from build123d import *

# Parameters (mm, degrees)
SZKIC1_R                    = 3
DODANIE_WYCI_GNI_CIE1_DEPTH = 2


with BuildPart() as part:
    # Szkic1 → Dodanie-wyciągnięcie1 (new body)
    with BuildSketch(Plane.XY):
        with BuildLine():
            ThreePointArc((16.690895301, 15.0061262), (12.690895301, 19.0061262), (8.690895301, 15.0061262))
            Line((8.690895301, 15.0061262), (6.71006463, -34.514640573))
            Line((6.71006463, -34.514640573), (6.690895301, -34.9938738))
            ThreePointArc((6.690895301, -34.9938738), (12.690895301, -40.9938738), (18.690895301, -34.9938738))
            Line((18.690895301, -34.9938738), (18.671725971, -34.514640573))
            Line((18.671725971, -34.514640573), (16.690895301, 15.0061262))
        make_face()
        with Locations((12.690895301, -34.9938738)):
            Circle(SZKIC1_R, mode=Mode.SUBTRACT)
        with Locations((12.690895301, 15.0061262)):
            Circle(SZKIC1_R, mode=Mode.SUBTRACT)
    extrude(amount=DODANIE_WYCI_GNI_CIE1_DEPTH)


solid = part.part
Verification items for the finished model (mm, model axes). Coordinates: 2 decimals unless noted, no trailing zeros. Order: outer loops, then holes, each group sorted by start corner. A loop starts at its lowest first (then second) coordinate and runs counter-clockwise, first axis right, second up. Notation, with made-up numbers: M -10.5,63 L 25.5,63 A22 ccw 25.5,85 Z; hole C 57,29 d4. An arc over 180 degrees is marked long. One line per item, written item: value. Start each with the question number.
Item 1: Depth check by flat-ended pin: P1, Ø7, axis at x = 12.69, y = 15.01, coming from the +Z side. Enter the tip coordinate at first touch or a pass-through.
Item 2: Sectioned sample at B-B on x = 12.75. Record the cut outline in (y, z).
Item 3: Thickness scan on probe 1 along Y at (x, z) = (12.5, 0.9); probe 2 along Y at (x, z) = (13.5, 1.25); probe 3 along X at (y, z) = (16, 0.6). Record the ranges inside material, lowest first.
Item 4: Sectioned sample at D-D on y = 10.5. Record the cut outline in (x, z).
Item 5: Sectioned sample at A-A on z = 1.6. Record the cut outline in (x, y), then the cut area to 3 significant figures.
Item 6: Mould release check, pull along Y, two halves, no side actions. Record for faces 1 (the flat face through (13, -17, 2)), 2 (the cylindrical face through (14.3, 17.54, 0.99)), 3 (the cylindrical face through (12.779, 19.005, 0.986)), 4 (the cylindrical face through (12.559, -40.992, 0.986)): pulls with the +Y half, pulls with the -Y half, needs draft (parallel to the pull), parting line crosses it, or undercut.
Item 7: Sectioned sample at C-C on y = -17. Record the cut outline in (x, z), then the cut area to 3 significant figures.
Calculated:
1. P1: z = 2
2. outline: M -40.99,0 L -37.99,0 L -37.99,2 L -40.99,2 Z; M -31.99,0 L 12.01,0 L 12.01,2 L -31.99,2 Z; M 18.01,0 L 19.01,0 L 19.01,2 L 18.01,2 Z
3. probe 1: -40.99 to -37.99, -32 to 12.01, 18 to 19
3. probe 2: -40.94 to -37.88, -32.11 to 12.12, 17.89 to 18.92
3. probe 3: 8.82 to 9.86, 15.52 to 16.57
4. outline: M 8.51,0 L 16.87,0 L 16.87,2 L 8.51,2 Z
5. outline: M 6.69,-34.99 A6 ccw 18.69,-34.99 L 16.69,15.01 A4 ccw 8.69,15.01 Z; hole C 12.69,-34.99 d6; hole C 12.69,15.01 d6
5. area: 525 mm^2
6. face 1: needs draft
6. face 2: undercut
6. face 3: pulls with the +Y half
6. face 4: pulls with the -Y half
7. outline: M 7.41,0 L 17.97,0 L 17.97,2 L 7.41,2 Z
7. area: 21.1 mm^2
